Autodesk Inventor part; units mm, degrees
ref_plane "YZ Plane" through (0, 0, 0) normal (1, 0, 0) x (0, 1, 0)
ref_plane "XZ Plane" through (0, 0, 0) normal (0, 1, 0) x (-1, 0, 0)
ref_plane "XY Plane" through (0, 0, 0) normal (0, 0, 1) x (1, 0, 0)
sketch "Sketch1" plane through (0, 0, 0) normal (0, 0, 1) x (1, 0, 0)
  line L0 (0, 0) -> (6.35, 0)
  line L1 (6.35, 0) -> (6.35, 12.7)
  line L2 (6.35, 12.7) -> (25.4, 12.7)
  line L3 (25.4, 12.7) -> (25.4, 0)
  line L4 (25.4, 0) -> (31.75, 0)
  circle A0 centre (15.875, 25.4) radius 4.7816
  line L5 (-32.385, 142.875) -> (-32.385, 111.125)
  line L6 (-32.385, 142.875) -> (22.225, 142.875)
  line L7 (31.75, 38.1) -> (0, 38.1) construction
  line L8 (53.975, -44.5659) -> (53.975, 161.925) construction
  line L9 (0, 38.1) -> (22.225, 63.5)
  line L10 (53.975, 63.5) -> (53.975, 161.925)
  line L11 (0, 0) -> (0, 38.1)
  line L12 (31.75, 0) -> (38.1, 0)
  line L13 (38.1, 0) -> (38.1, 38.1)
  line L14 (38.1, 38.1) -> (53.975, 63.5)
  line L15 (53.975, 63.5) -> (53.975, 161.925)
  line L16 (22.225, 63.5) -> (22.225, 142.875)
  line L17 (-32.385, 142.875) -> (22.225, 142.875)
  line L18 (0, 0) -> (0, 38.1)
  line L19 (0, 38.1) -> (22.225, 63.5)
  line L20 (22.225, 63.5) -> (22.225, 142.875)
  line L21 (22.225, 142.875) -> (-32.385, 142.875)
  line L22 (-32.385, 142.875) -> (-32.385, 111.125)
  line L23 (6.35, 12.7) -> (25.4, 12.7)
  line L24 (25.4, 12.7) -> (25.4, 0)
  line L25 (38.1, 0) -> (25.4, 0)
  line L26 (38.1, 0) -> (38.1, 38.1)
  line L27 (53.975, 63.5) -> (38.1, 38.1)
  line L28 (53.975, 63.5) -> (53.975, 161.925)
  line L29 (38.1, 0) -> (25.4, 0)
  line L30 (-63.5, -52.3717) -> (-63.5, 366.3054) construction
  line L31 (-63.5, 142.875) -> (-63.5, 246.5917)
  line L32 (-63.5, 246.5917) -> (-44.45, 246.5917)
  line L33 (-32.385, 111.125) -> (-63.5, 142.875)
  line L34 (-44.45, 246.5917) -> (53.975, 161.925)
  line L35 (-41.91, 161.925) -> (34.5004, 161.925)
  line L36 (34.5004, 161.925) -> (-41.91, 227.6544)
  line L37 (-41.91, 161.925) -> (-41.91, 227.6544)
  dimension "d0" = 6.35
  dimension "d1" = 12.7
  dimension "d2" = 19.05
  dimension "d3" = 6.35
  dimension "d5" = 9.5631
  dimension "d6" = 12.7
  dimension "d7" = 9.525
  dimension "d11" = 31.75
  dimension "d23" = 25.4
  dimension "d24" = 38.1
  dimension "d25" = 25.4
  dimension "d26" = 38.1
  dimension "d27" = 54.61
  dimension "d32" = 6.35
  dimension "d33" = 22.225
  dimension "d34" = 38.1
  dimension "d36" = 79.375
  dimension "d60" = 117.475
  dimension "d61" = 103.7167
  dimension "d62" = 19.05
  dimension "d64" = 31.75
  dimension "d66" = 31.115
  dimension "d88" = 12.7
  dimension "d89" = 40.703
  dimension "d91" = 21.59
  dimension "d92" = 19.05
ref_plane "Work Plane1" through (0, 0, 9.525) normal (0, 0, 1) x (1, 0, 0)
ref_plane "Work Plane2" through (0, 0, 9.525) normal (0, 0, 1) x (1, 0, 0)
extrude "Extrusion6" add sketch "Sketch1" along normal blind 6.35
sketch "Sketch5" plane through (0, 0, 6.35) normal (0, 0, 1) x (1, 0, 0)
  line L0 (-44.45, 246.5917) -> (-63.5, 246.5917)
  line L1 (-63.5, 246.5917) -> (-63.5, 142.875)
  circle A0 centre (-47.3583, 218.3215) radius 1.905
  circle A1 centre (-57.4675, 195.3091) radius 1.905
  dimension "d95" = 3.81
  dimension "d96" = 3.81
  dimension "d97" = 28.2702
  dimension "d98" = 51.2826
  dimension "d99" = 6.0325
  dimension "d100" = 16.1417
extrude "Extrusion7" cut sketch "Sketch5" against normal blind 9.525
fillet "Fillet3" radius 3.175 16 edges at (-44.45, 246.5917, 3.175) (-63.5, 246.5917, 3.175) (53.975, 161.925, 3.175) (-41.91, 161.925, 3.175) (53.975, 63.5, 3.175) (38.1, 38.1, 3.175) (38.1, 0, 3.175) (0, 0, 3.175) (0, 38.1, 3.175) (22.225, 63.5, 3.175) (22.225, 142.875, 3.175) (-32.385, 111.125, 3.175) (-63.5, 142.875, 3.175) (-32.385, 142.875, 3.175) (-41.91, 227.6544, 3.175) (34.5004, 161.925, 3.175)
sketch "Sketch6" plane through (0, 0, 6.35) normal (0, 0, 1) x (1, 0, 0)
  line L0 (-29.21, 142.875) -> (19.05, 142.875)
  line L1 (25.9409, 161.925) -> (-38.735, 161.925)
  circle A0 centre (-25.4, 155.575) radius 1.5875
  circle A1 centre (-25.4, 147.6375) radius 1.5875
  line L2 (-63.5, 243.4167) -> (-63.5, 144.1714)
  point P0 (0, 0)
  dimension "d104" = 3.175
  dimension "d105" = 3.175
  dimension "d106" = 4.7625
  dimension "d107" = 6.35
  dimension "d110" = 38.1
  dimension "d111" = 38.1
extrude "Extrusion8" cut sketch "Sketch6" against normal blind 9.525
sketch "Sketch7" plane through (0, 0, 6.35) normal (0, 0, 1) x (1, 0, 0)
  line L0 (-29.21, 142.875) -> (19.05, 142.875)
  line L1 (22.225, 139.7) -> (22.225, 64.693)
  line L2 (-44.45, 165.1) -> (-44.45, 222.9201)
  line L3 (122.6353, 104.775) -> (-142.2483, 104.775) construction
  circle A0 centre (38.354, 101.6) radius 1.905
  circle A1 centre (28.2448, 78.5876) radius 1.905
  point P0 (0, 0)
  dimension "d112" = 38.1
  dimension "d113" = 3.81
  dimension "d114" = 3.81
  dimension "d115" = 23.0124
  dimension "d116" = 10.1092
  dimension "d117" = 6.0198
  dimension "d118" = 3.175
extrude "Extrusion9" cut sketch "Sketch7" against normal blind 9.525
properties part number "Bent Right Hook" material "Aluminum 6061"
Source: CAD feature listing. Evaluate the final solid. Frame: model axes, mm. A direction names the side the tool comes from. Round coordinates to 2 decimals unless told otherwise and drop trailing zeros. Loops run counter-clockwise (first coordinate to the right, second up) from the corner with the lowest first, then second, coordinate; pieces in that order, holes last.
1. Ray query, L1, parallel to Y at x = 14.5, z = 1 (3 decimals); L2, parallel to Y at x = 21, z = 1.5 (3 decimals); L3, parallel to X at y = 101.6, z = 3.75 (3 decimals). Return the intervals inside material, ascending.
2. Section query B-B on x = -14. Output: boundary loops of the cut face in (y, z) (3 decimals), and give its area (3 significant figures).
3. Section query C-C on z = 5. Give the number of separate pieces and of enclosed holes in the cut face, and give its area (3 significant figures).
4. Access query for faces 5 (the flat face through (22.225, 102, 3)), 6 (the flat face through (10.968, 50.635, 3.131)), 7 (the flat face through (-63.5, 193, 3)), 8 (the flat face through (6.35, 6, 3)), 9 (the flat face through (0, 20, 3)). Directions: +Z, -Z, +X, -X, +Y, -Y. A direction counts if a zero-diameter tool reaches every point of the face in a straight line with its end or side. Return the directions, or none.
5. Section query A-A on y = 25.4. Output: boundary loops of the cut face in (x, z), and give its area (3 significant figures).
6. Contact query for flat-ended pins moving along their axis: pin 1 (1.9 mm diameter, centred on x = 17.5, z = 2.5, fed in from -Y); pin 2 (3 mm diameter, centred on y = 5, z = 2, fed in from +X); pin 3 (1.9 mm diameter, centred on x = -14, z = 4.5, fed in from +Y). Output: stop coordinate, or through.
7. Mould query, pull axis X, two halves, no side actions, for faces 1 (the flat face through (-53, 246.592, 3)), 2 (the flat face through (-50, 129.1, 3.1)), 3 (the flat face through (38.1, 20, 3)), 4 (the flat face through (-3.874, 194.935, 3.131)). Classes: released by +X, released by -X, zero draft, split by the parting line, or undercut.
Answers below:
1. L1: y = 12.7 to 20.82, 29.98 to 54.671, 142.875 to 161.925, 179.13 to 195.882
1. L2: y = 12.7 to 62.1, 142.206 to 161.925, 173.538 to 190.291
1. L3: x = 22.225 to 36.449, 40.259 to 53.975
2. outline: (142.875, 0) - (161.925, 0) - (161.925, 6.35) - (142.875, 6.35) - close; (203.646, 0) - (220.398, 0) - (220.398, 6.35) - (203.646, 6.35) - close
2. area: 227 mm2
3. separate pieces: 1
3. enclosed holes: 8
3. area: 10,500 mm2
4. face 5: +Z, -Z
4. face 6: +Z, -Z, -X
4. face 7: +Z, -Z, -X, +Y, -Y
4. face 8: +Z, -Z, -Y
4. face 9: +Z, -Z, -X, -Y
5. outline: (0, 0) - (11.09, 0) - (11.09, 6.35) - (0, 6.35) - close; (20.66, 0) - (38.1, 0) - (38.1, 6.35) - (20.66, 6.35) - close
5. area: 181 mm2
6. pin 1: stops at y = 12.7
6. pin 2: stops at x = 38.1
6. pin 3: stops at y = 221.22
7. face 1: zero draft
7. face 2: released by -X
7. face 3: released by +X
7. face 4: undercut
